Can you work these out from the model? Positions are in its coordinate system, mm. Face numbers are marked on the shaded views. A direction names the side the tool comes from. Give positions to 0.01 mm unless a question says otherwise; leave off trailing zeros. Order: outer loops, then holes, each group sorted by start corner. A loop starts at its lowest first (then second) coordinate and runs counter-clockwise, first axis right, second up. Notation, with made-up numbers: (1, 38) - (6, 38) arc R8 cw to (6, 46) - close; hole circle Ø5 at (12.5, -13.75). An arc over 180 degrees is marked (long way). Return JSON: item names as keys, results as strings.
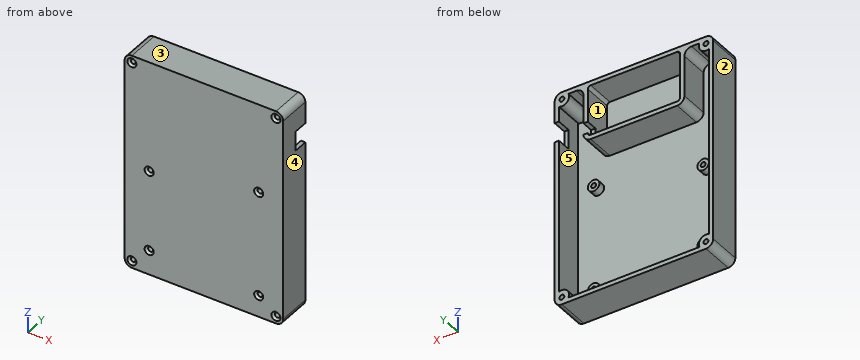
```python
from build123d import *

# Parameters (mm, degrees)
ESBO_O1_W                                            = 110
ESBO_O1_H                                            = 150
RESSALTO_EXTRUS_O3_DEPTH                             = 23
FILETE2_R                                            = 5
CASCA1_T                                             = -3
ESBO_O14_R                                           = 5
RESSALTO_EXTRUS_O7_DEPTH                             = 20
RESSALTO_EXTRUS_O4_DEPTH                             = 23
FILETE6_R                                            = 2
FILETE8_R                                            = 5
ESBO_O7_W                                            = 3
ESBO_O7_H                                            = 8
CORTE_EXTRUS_O1_DEPTH                                = 8
ESBO_O8_W                                            = 3
ESBO_O8_H                                            = 13.5
CORTE_EXTRUS_O2_DEPTH                                = 10
ESBO_O17_R                                           = 4
RESSALTO_EXTRUS_O8_DEPTH                             = 5
ESCAREADO_PARA_PARAFUSO_DE_M_QUINA_COM_C_D           = 3.4
ESCAREADO_PARA_PARAFUSO_DE_M_QUINA_COM_C_DEPTH       = 15
ESCAREADO_PARA_PARAFUSO_DE_M_QUINA_COM_C_CSINK_D     = 6.3
ESCAREADO_PARA_PARAFUSO_DE_M_QUINA_COM_C_CSINK_ANGLE = 90
ESCAREADO_PARA_PARAFUSO_DE_M_QUINA_COM_C_TIP         = 1.021463052
ESCAREADO_PARA_PARAFUSO_DE_M_QUINA_C_2_D             = 3.4
ESCAREADO_PARA_PARAFUSO_DE_M_QUINA_C_2_CSINK_D       = 6.3
ESCAREADO_PARA_PARAFUSO_DE_M_QUINA_C_2_CSINK_ANGLE   = 90


with BuildPart() as part:
    # Esboço1 → Ressalto-extrusão3 (new body)
    with BuildSketch(Plane(origin=(0, 0, 0), x_dir=(1, 0, 0), z_dir=(0, 1, 0))):
        Rectangle(ESBO_O1_W, ESBO_O1_H)
    extrude(amount=RESSALTO_EXTRUS_O3_DEPTH)

    # Filete2
    filete2_edges = [part.edges().sort_by_distance(p)[0] for p in [
        (55, 11.5, 75),
        (-55, 11.5, 75),
        (-55, 11.5, -75),
        (55, 11.5, -75),
    ]]
    fillet(filete2_edges, radius=FILETE2_R)

    # Casca1
    casca1_openings = [part.faces().sort_by_distance(p)[0] for p in [
        (0, 23, 0),
    ]]
    offset(amount=CASCA1_T, openings=casca1_openings, kind=Kind.INTERSECTION)

    # Esboço14 → Ressalto-extrusão7 (add)
    with BuildSketch(Plane(origin=(0, 3, 0), x_dir=(1, 0, 0), z_dir=(0, 1, 0))):
        with Locations((-50, -70)):
            Circle(ESBO_O14_R)
        with Locations((50, -70)):
            Circle(ESBO_O14_R)
        with Locations((50, 70)):
            Circle(ESBO_O14_R)
        with Locations((-50, 70)):
            Circle(ESBO_O14_R)
    extrude(amount=RESSALTO_EXTRUS_O7_DEPTH)

    # Esboço6 → Ressalto-extrusão4 (add)
    with BuildSketch(Plane(origin=(0, 0, 0), x_dir=(1, 0, 0), z_dir=(0, 1, 0))):
        Polygon((-32, -37), (32, -37), (32, -72), (35, -72), (35, -34), (-35, -34), (-35, -72), (-32, -72), align=None)
    extrude(amount=RESSALTO_EXTRUS_O4_DEPTH)

    # Filete6
    filete6_edges = [part.edges().sort_by_distance(p)[0] for p in [
        (32, 13, 37),
        (-32, 13, 37),
        (-32, 13, 72),
        (32, 13, 72),
    ]]
    fillet(filete6_edges, radius=FILETE6_R)

    # Filete8
    filete8_edges = [part.edges().sort_by_distance(p)[0] for p in [
        (-35, 13, 72),
        (-35, 13, 34),
        (35, 13, 34),
        (35, 13, 72),
    ]]
    fillet(filete8_edges, radius=FILETE8_R)

    # Esboço7 → Corte-extrusão1 (cut)
    with BuildSketch(Plane(origin=(0, 23, 0), x_dir=(1, 0, 0), z_dir=(0, 1, 0))):
        with Locations((33.5, -43)):
            Rectangle(ESBO_O7_W, ESBO_O7_H)
    extrude(amount=-CORTE_EXTRUS_O1_DEPTH, mode=Mode.SUBTRACT)

    # Esboço8 → Corte-extrusão2 (cut)
    with BuildSketch(Plane(origin=(0, 23, 0), x_dir=(1, 0, 0), z_dir=(0, 1, 0))):
        with Locations((53.5, -48.25)):
            Rectangle(ESBO_O8_W, ESBO_O8_H)
    extrude(amount=-CORTE_EXTRUS_O2_DEPTH, mode=Mode.SUBTRACT)

    # Esboço17 → Ressalto-extrusão8 (add)
    with BuildSketch(Plane(origin=(0, 3, 0), x_dir=(1, 0, 0), z_dir=(0, 1, 0))):
        with Locations((-38, 58)):
            Circle(ESBO_O17_R)
        with Locations((-38, 2)):
            Circle(ESBO_O17_R)
        with Locations((38, -13)):
            Circle(ESBO_O17_R)
        with Locations((38, 60)):
            Circle(ESBO_O17_R)
    extrude(amount=RESSALTO_EXTRUS_O8_DEPTH)

    # Escareado para parafuso de m_quina com c
    with Locations(Plane(origin=(0, 0, 0), x_dir=(-1, 0, 0), z_dir=(0, -1, 0))):
        with Locations((-38, -13), (38, 2), (38, 58), (-38, 60)):
            CounterSinkHole(ESCAREADO_PARA_PARAFUSO_DE_M_QUINA_COM_C_D / 2, ESCAREADO_PARA_PARAFUSO_DE_M_QUINA_COM_C_CSINK_D / 2, depth=ESCAREADO_PARA_PARAFUSO_DE_M_QUINA_COM_C_DEPTH, counter_sink_angle=ESCAREADO_PARA_PARAFUSO_DE_M_QUINA_COM_C_CSINK_ANGLE)
            with Locations((0, 0, -(ESCAREADO_PARA_PARAFUSO_DE_M_QUINA_COM_C_DEPTH + ESCAREADO_PARA_PARAFUSO_DE_M_QUINA_COM_C_TIP / 2))):  # 118° drill point
                Cone(0, ESCAREADO_PARA_PARAFUSO_DE_M_QUINA_COM_C_D / 2, ESCAREADO_PARA_PARAFUSO_DE_M_QUINA_COM_C_TIP, mode=Mode.SUBTRACT)

    # Escareado para parafuso de m_quina c 2 (through all)
    with Locations(Plane(origin=(0, 0, 0), x_dir=(-1, 0, 0), z_dir=(0, -1, 0))):
        with Locations((50, -70), (-50, -70), (-50, 70), (50, 70)):
            CounterSinkHole(ESCAREADO_PARA_PARAFUSO_DE_M_QUINA_C_2_D / 2, ESCAREADO_PARA_PARAFUSO_DE_M_QUINA_C_2_CSINK_D / 2, counter_sink_angle=ESCAREADO_PARA_PARAFUSO_DE_M_QUINA_C_2_CSINK_ANGLE)


solid = part.part
```
1. Thinking about a two-plate mould opening in X: for the marked faces 3, 4 and 5, which applies, +X half, -X half, draft (parallel to the pull), parting line (faces both ways), or undercut?
Checks:
{"face 3": "draft", "face 4": "+X half", "face 5": "undercut"}
2. Suppose I cut it at C-C (z = 28). List the corners of the cut face in (x, y) for me, plus the area to 3 significant figures.
Checks:
{"outline": "(-55, 0) - (55, 0) - (55, 23) - (52, 23) - (52, 3) - (-52, 3) - (-52, 23) - (-55, 23) - close", "area": "450 mm^2"}
3. On a 3-axis mill with a long thin cutter (end or side, diameter ignored), from which of +Z, -Z, +X, -X, +Y, -Y can I reach the whole of each face in a straight line? I mean the marked faces 1 and 2. Say none if no direction works.
Checks:
{"face 1": "+Y", "face 2": "+Z, -Z, -X, +Y, -Y"}
4. Suppose I cut it at B-B (x = -38). List the corners of the cut face in (y, z) for me.
Checks:
{"outline": "(0, -75) - (23, -75) - (23, -72) - (3, -72) - (3, -62) - (8, -62) - (8, -59.7) - (1.45, -59.7) - (0, -61.15) - close; (0, -54.85) - (1.45, -56.3) - (8, -56.3) - (8, -54) - (3, -54) - (3, -6) - (8, -6) - (8, -3.7) - (1.45, -3.7) - (0, -5.15) - close; (0, 1.15) - (1.45, -0.3) - (8, -0.3) - (8, 2) - (3, 2) - (3, 71.58) - (23, 71.58) - (23, 75) - (0, 75) - close"}
5. For pin 1 Ø6 at (x, z) = (-27.5, -50) entering from +Y; pin 2 Ø2 at (x, z) = (38, 13) entering from -Y; pin 3 Ø3.5 at (x, z) = (53, 49.5) entering from +Y; pin 4 Ø4 at (x, z) = (38, -60) entering from -Y, each with a flat end and sliding along its axis, tell me the tip position at first contact or that it passes through.
Checks:
{"pin 1": "y = 3", "pin 2": "through", "pin 3": "y = 13", "pin 4": "y = 1.15"}
6. Suppose I cut it at D-D (x = 1.5). List the corners of the cut face in (y, z) for me, plus the area to 3 significant figures.
Checks:
{"outline": "(0, -75) - (23, -75) - (23, -72) - (3, -72) - (3, 34) - (23, 34) - (23, 37) - (3, 37) - (3, 72) - (23, 72) - (23, 75) - (0, 75) - close", "area": "630 mm^2"}
7. Suppose I cut it at A-A (z = 13). List the corners of the cut face in (x, y) for me, plus the area to 3 significant figures.
Checks:
{"outline": "(-55, 0) - (34.85, 0) - (36.3, 1.45) - (36.3, 8) - (34, 8) - (34, 3) - (-52, 3) - (-52, 23) - (-55, 23) - close; (39.7, 1.45) - (41.15, 0) - (55, 0) - (55, 23) - (52, 23) - (52, 3) - (42, 3) - (42, 8) - (39.7, 8) - close", "area": "461 mm^2"}
8. If I drill on L1, parallel to X at y = 8.5, z = 46; L2, parallel to Z at x = -50, y = 9.5; L3, parallel to Z at x = 29, y = 9.25, over which ranges is the centre line in solid material (lowest first)? Write a range as [from, to].
Checks:
{"L1": "[-55, -52], [-35, -32], [32, 35], [52, 55]", "L2": "[-75, -71.7], [-68.3, -65], [65, 68.3], [71.7, 75]", "L3": "[-75, -72], [34, 37], [72, 75]"}
